```python
from build123d import *

# Parameters (mm, degrees)
EXTRUDE_F_DEPTH    = 1016
CUT_EXTRUDE1_DEPTH = 3.175


with BuildPart() as part:
    # Sketch1 → Extrude f (new body)
    with BuildSketch(Plane.XY):
        Polygon((3.175, 3.175), (3.175, 12.7), (0, 12.7), (0, 0), (38.1, 0), (38.1, 12.7), (34.925, 12.7), (34.925, 3.175), align=None)
    extrude(amount=EXTRUDE_F_DEPTH)

    # Sketch2 → Cut-Extrude1 (cut)
    with BuildSketch(Plane(origin=(0, 3.175, 0), x_dir=(1, 0, 0), z_dir=(0, 1, 0))):
        with BuildLine():
            Line((6.35, -952.5), (6.35, -876.3))
            ThreePointArc((6.35, -876.3), (19.05, -863.6), (31.75, -876.3))
            Line((31.75, -876.3), (31.75, -952.5))
            ThreePointArc((31.75, -952.5), (19.05, -965.2), (6.35, -952.5))
        make_face()
    cut_extrude1 = extrude(amount=-CUT_EXTRUDE1_DEPTH, mode=Mode.SUBTRACT)

    # Mirror1: Cut-Extrude1 across plane
    add(cut_extrude1.mirror(Plane.XY.offset(508)), mode=Mode.SUBTRACT)


solid = part.part
```
Check sheet for the modelled part. Datum: model origin and axes. Units: mm. Coordinates: 2 decimals unless noted, no trailing zeros. Write each loop counter-clockwise with the first axis right and the second up, starting at its lowest first coordinate (ties: lowest second). Pieces come first, ordered by that corner, then holes. Notation, with made-up numbers: (-9, -28) -> (22, -28) arc R16 cw to (22, -23) -> close; hole circle Ø5 at (40.25, 42.25). An arc over 180 degrees is marked (long way). Use a Markdown table: item, result.
1. Sectioned sample at C-C (x = 19.05). Enter the section's corners in (y, z) (3 decimals), plus the area to 3 significant figures.
Reported:
| item | result |
|---|---|
| outline | (0, 0) -> (3.175, 0) -> (3.175, 50.8) -> (0, 50.8) -> close; (0, 152.4) -> (3.175, 152.4) -> (3.175, 863.6) -> (0, 863.6) -> close; (0, 965.2) -> (3.175, 965.2) -> (3.175, 1016) -> (0, 1016) -> close |
| area | 2,580 mm2 |
2. Scan lines: line 1 along X through (y, z) = (9.25, 408) (3 decimals); line 2 along Y through (x, z) = (5.5, 259) (3 decimals); line 3 along X through (y, z) = (1, 59.5). Record each from-to range of solid material in increasing order.
Reported:
| item | result |
|---|---|
| line 1 | x = 0 to 3.175, 34.925 to 38.1 |
| line 2 | y = 0 to 3.175 |
| line 3 | x = 0 to 7, 31.1 to 38.1 |
3. Sectioned sample at D-D (z = 281.5). Enter the section's corners in (x, y) (3 decimals), plus the area to 3 significant figures.
Reported:
| item | result |
|---|---|
| outline | (0, 0) -> (38.1, 0) -> (38.1, 12.7) -> (34.925, 12.7) -> (34.925, 3.175) -> (3.175, 3.175) -> (3.175, 12.7) -> (0, 12.7) -> close |
| area | 181 mm2 |
4. Release check for a two-part mould opening along X. For faces 1 (the flat face through (19, 0, 501)), 2 (the flat face through (19, 3.175, 501)) record: pulls with the +X half, pulls with the -X half, needs draft (parallel to the pull), parting line crosses it, or undercut.
Reported:
| item | result |
|---|---|
| face 1 | needs draft |
| face 2 | undercut |
5. Sectioned sample at A-A (z = 907). Enter the section's corners in (x, y) (3 decimals).
Reported:
| item | result |
|---|---|
| outline | (0, 0) -> (6.35, 0) -> (6.35, 3.175) -> (3.175, 3.175) -> (3.175, 12.7) -> (0, 12.7) -> close; (31.75, 0) -> (38.1, 0) -> (38.1, 12.7) -> (34.925, 12.7) -> (34.925, 3.175) -> (31.75, 3.175) -> close |
6. Go/stop test with a flat-tipped pin: pin 1 Ø16 at (x, z) = (20.5, 559.5) entering from +Y (3 decimals). Record where the tip stops, or that it passes through.
Reported:
| item | result |
|---|---|
| pin 1 | stops at y = 3.175 |
7. Sectioned sample at B-B (y = 8.25). Enter the section's corners in (x, z) (3 decimals), plus the area to 3 significant figures.
Reported:
| item | result |
|---|---|
| outline | (0, 0) -> (3.175, 0) -> (3.175, 1016) -> (0, 1016) -> close; (34.925, 0) -> (38.1, 0) -> (38.1, 1016) -> (34.925, 1016) -> close |
| area | 6,450 mm2 |
